The listing builds one solid part. Answer for the finished solid, in the listing's coordinates (mm). A direction names the side the tool comes from. Round coordinates to 2 decimals unless told otherwise and drop trailing zeros. Write each loop counter-clockwise with the first axis right and the second up, starting at its lowest first coordinate (ties: lowest second). Pieces come first, ordered by that corner, then holes.
Item 1: Find section B-B on x = 53. Give the number of separate pieces and of enclosed holes in the cut face, then the cut area to 3 significant figures.
Item 2: Each of these flat-tipped pins is pushed along its axis until it touches: pin 1 (1 mm diameter, centred on x = 97, z = 2, fed in from +Y); pin 2 (8 mm diameter, centred on y = 22, z = -38.5, fed in from +X); pin 3 (10 mm diameter, centred on x = -76.5, y = 101.5, fed in from +Z); pin 4 (19 mm diameter, centred on x = -50.65, y = -29.24, fed in from -Z). Where does it stop, or does it pass through?
Item 3: For a pull along X with two mould halves and no side action, classify faces 1 (the face through (-81, -71, 40)), 2 (the face through (20, -20, -10)), 3 (the face through (-78.637, -72.108, 41.972)) as +X half, -X half, draft (parallel to the pull), parting line (faces both ways), or undercut.
Item 4: Find the intervals of material crossed by probe 1 along Y at (x, z) = (47, 5); probe 2 along Y at (x, z) = (0, 35); probe 3 along Y at (x, z) = (-70.5, -30.5), in increasing order.
Item 5: Find section C-C on z = -34. Give the vertices of the cut face in (x, y), then the cut area to 3 significant figures.
Item 6: A tool of negligible diameter and unlimited length cuts with its end or side. For faces 4 (the face through (20, -20, 10)), 5 (the face through (-18.15, -13.91, 0.14)), 6 (the face through (89.336, 28.133, -29.72)), from which of +Z, -Z, +X, -X, +Y, -Y can it reach the whole face along a straight path? Write none if from no direction.
Autodesk Inventor part; units mm, degrees
ref_plane "YZ Plane" through (0, 0, 0) normal (1, 0, 0) x (0, 1, 0)
ref_plane "XZ Plane" through (0, 0, 0) normal (0, 1, 0) x (-1, 0, 0)
ref_plane "XY Plane" through (0, 0, 0) normal (0, 0, 1) x (1, 0, 0)
sketch "Sketch1" plane through (0, 0, 0) normal (0, 0, 1) x (1, 0, 0)
  circle A0 centre (0, 0) radius 150
  circle A1 centre (0, 0) radius 106.693
  dimension "d0" = 300
extrude "Extrusion1" add sketch "Sketch1" along normal mid plane 80
fillet "Fillet1" radius 30 2 edges at (-150, 0, 40) (-150, 0, -40)
sketch "Sketch2" plane through (0, 0, 0) normal (0, 0, 1) x (1, 0, 0)
  circle A0 centre (0, 0) radius 106.693
  circle A1 centre (0, 0) radius 93.6614
extrude "Extrusion2" add sketch "Sketch2" along normal mid plane 100
fillet "Fillet2" radius 6 2 edges at (-106.693, 0, -50) (-106.693, 0, 50)
sketch "Sketch3" plane through (0, 0, 0) normal (0, 0, 1) x (1, 0, 0)
  circle A0 centre (0, 0) radius 93.6614
  circle A1 centre (0, 0) radius 22.8659
  circle A2 centre (0, 58.4849) radius 11.9417
  circle A3 centre (-50.6494, 29.2425) radius 11.9417
  circle A4 centre (-50.6494, -29.2425) radius 11.9417
  circle A5 centre (0, -58.4849) radius 11.9417
  circle A6 centre (50.6494, -29.2425) radius 11.9417
  circle A7 centre (50.6494, 29.2425) radius 11.9417
  dimension "d9" = 360
extrude "Extrusion3" add sketch "Sketch3" along normal mid plane 20
properties part number "rear"
Check values:
1. separate pieces: 3
1. enclosed holes: 0
1. area: 12,000 mm2
2. pin 1: stops at y = 114.84
2. pin 2: stops at x = 135.58
2. pin 3: stops at z = 39.93
2. pin 4: passes through
3. face 1: draft
3. face 2: undercut
3. face 3: parting line
4. probe 1: y = -142.45 to -40.61, -17.87 to 17.87, 40.61 to 142.45
4. probe 2: y = -136.58 to -93.66, 93.66 to 136.58
4. probe 3: y = -123.15 to -61.66, 61.66 to 123.15
5. outline: circle Ø276 at (0, 0); hole circle Ø187.32 at (0, 0)
5. area: 32,300 mm2
6. face 4: +Z
6. face 5: +Z, -Z
6. face 6: -Z
